Design review of the part built by this model. Coordinates are the model's own, in mm. A direction names the side the tool comes from. Give positions to 0.01 mm unless a question says otherwise; leave off trailing zeros. Loops run counter-clockwise (first coordinate to the right, second up) from the corner with the lowest first, then second, coordinate; pieces in that order, holes last. Notation, with made-up numbers: (13, -9.5) - (47, -9.5) arc R19 ccw to (47, 2.5) - close; hole circle Ø9 at (34.25, -24). An arc over 180 degrees is marked (long way). Write each question's results on one line, items separated by ' | '.
from build123d import *

# Parameters (mm, degrees)
SKETCH_1_R      = 2
EXTRUDE_1_DEPTH = 3


with BuildPart() as part:
    # 草圖1 → 填料-伸長1 (new body)
    with BuildSketch(Plane.XY):
        with BuildLine():
            Line((59.29779344, 4.218826045), (27.815049638, 66.504924261))
            ThreePointArc((27.815049638, 66.504924261), (22.280452319, 71.817413106), (14.658767156, 72.691610154))
            Line((14.658767156, 72.691610154), (-41.535085268, 59.909886888))
            ThreePointArc((-41.535085268, 59.909886888), (-64.065081782, 42.747842637), (-66.156088343, 14.503122823))
            Line((-66.156088343, 14.503122823), (-44.645241189, -44.597442609))
            Line((-44.645241189, -44.597442609), (-37.145243156, -44.597442609))
            Line((-37.145243156, -44.597442609), (-37.145243156, -59.597442609))
            Line((-37.145243156, -59.597442609), (31.854756844, -59.597442609))
            Line((31.854756844, -59.597442609), (31.854756844, -44.597442609))
            Line((31.854756844, -44.597442609), (39.352422835, -44.597442609))
            Line((39.352422835, -44.597442609), (57.472801714, -29.392639375))
            ThreePointArc((57.472801714, -29.392639375), (59.36662348, -26.84637358), (60.037958839, -23.74486762))
            Line((60.037958839, -23.74486762), (60.037958839, 0.970036375))
            ThreePointArc((60.037958839, 0.970036375), (59.850576653, 2.636055511), (59.29779344, 4.218826045))
        make_face()
        with Locations((17.869885774, 62.635186946)):
            Circle(SKETCH_1_R, mode=Mode.SUBTRACT)
        with Locations((-2.073498249, 11.257790191)):
            Circle(SKETCH_1_R, mode=Mode.SUBTRACT)
        with Locations((-7.872108914, 3.110636432)):
            Circle(SKETCH_1_R, mode=Mode.SUBTRACT)
        with Locations((-41.668665513, 39.439038022)):
            Circle(SKETCH_1_R, mode=Mode.SUBTRACT)
        with Locations((-47.467276178, 31.291884264)):
            Circle(SKETCH_1_R, mode=Mode.SUBTRACT)
        Polygon((-40.901751655, 32.756086344), (-46.700362319, 24.608932586), (-14.111747287, 1.414489926), (-2.514525958, 17.708797442), (-35.10314099, 40.903240102), align=None, mode=Mode.SUBTRACT)
    extrude(amount=EXTRUDE_1_DEPTH)


solid = part.part
(1) Take a section at A-A on x = -25.5. Give the boundary of the cut face in (y, z).
Answers below:
outline: (-59.6, 0) - (9.52, 0) - (9.52, 3) - (-59.6, 3) - close; (34.07, 0) - (63.56, 0) - (63.56, 3) - (34.07, 3) - close
(2) Wall thickness on line 1 along X through (y, z) = (38, 1.65); line 2 along X through (y, z) = (24.5, 0.2); line 3 along Y through (x, z) = (-17, 2.3): over which ranges is each line inside the solid? List them lowest first. Write a range as from..to.
Answers below:
line 1: -66.19..-43.06, -40.28..-37.17, -31.02..42.22 | line 2: -68.19..-46.55, -12.06..49.05 | line 3: -59.6..3.47, 28.02..65.49
(3) Tool access review of faces 4 (the flat face through (36, -44.597, 1)), 5 (the flat face through (-37.145, -52, 1)), 6 (the flat face through (-30.63, 13.17, 1.48)): name each direction out of +Z, -Z, +X, -X, +Y, -Y from which nothing blocks a thin tool from reaching the whole face with its end or side.
Answers below:
face 4: +Z, -Z, +X, -Y | face 5: +Z, -Z, -X, -Y | face 6: +Z, -Z
(4) Take a section at D-D on y = 52.5. Give the boundary of the cut face in (x, z).
Answers below:
outline: (-56.19, 0) - (34.89, 0) - (34.89, 3) - (-56.19, 3) - close
(5) Draft analysis for pull direction Y (two halves, no side actions). For faces 1 (the flat face through (-55.551, -14.633, 1.479)), 2 (the cylindrical face through (59.856, 2.613, 1.479)), 3 (the cylindrical face through (-9.459, 1.894, 1.479)), state which applies: pulls with the +Y half, pulls with the -Y half, needs draft (parallel to the pull), parting line crosses it, or undercut.
Answers below:
face 1: pulls with the -Y half | face 2: pulls with the +Y half | face 3: undercut
(6) Take a section at B-B on z = 1.05. Give the boundary of the cut face in (x, y), plus the area to 3 significant figures.
Answers below:
outline: (-66.16, 14.5) - (-44.65, -44.6) - (-37.15, -44.6) - (-37.15, -59.6) - (31.85, -59.6) - (31.85, -44.6) - (39.35, -44.6) - (57.47, -29.39) arc R7.5 ccw to (60.04, -23.74) - (60.04, 0.97) arc R7.5 ccw to (59.3, 4.22) - (27.82, 66.5) arc R12 ccw to (14.66, 72.69) - (-41.54, 59.91) arc R34.5 ccw to start; hole circle Ø4 at (-47.47, 31.29); hole (-46.7, 24.61) - (-14.11, 1.41) - (-2.51, 17.71) - (-35.1, 40.9) - close; hole circle Ø4 at (-41.67, 39.44); hole circle Ø4 at (-7.87, 3.11); hole circle Ø4 at (-2.07, 11.26); hole circle Ø4 at (17.87, 62.64) | area: 12,100 mm2
(7) Insertion check: P1, Ø1.5, axis at y = -54, z = 2, coming from the +X side; P2, Ø1.5, axis at y = -52, z = 1.5, coming from the -X side. Each pin has a flat end and moves straight along its axis. Give the tip position at first contact, or say it passes through.
Answers below:
P1: x = 31.85 | P2: x = -37.15
(8) Take a section at C-C on x = 17.5. Give the boundary of the cut face in (y, z).
Answers below:
outline: (-59.6, 0) - (60.67, 0) - (60.67, 3) - (-59.6, 3) - close; (64.6, 0) - (72.95, 0) - (72.95, 3) - (64.6, 3) - close
